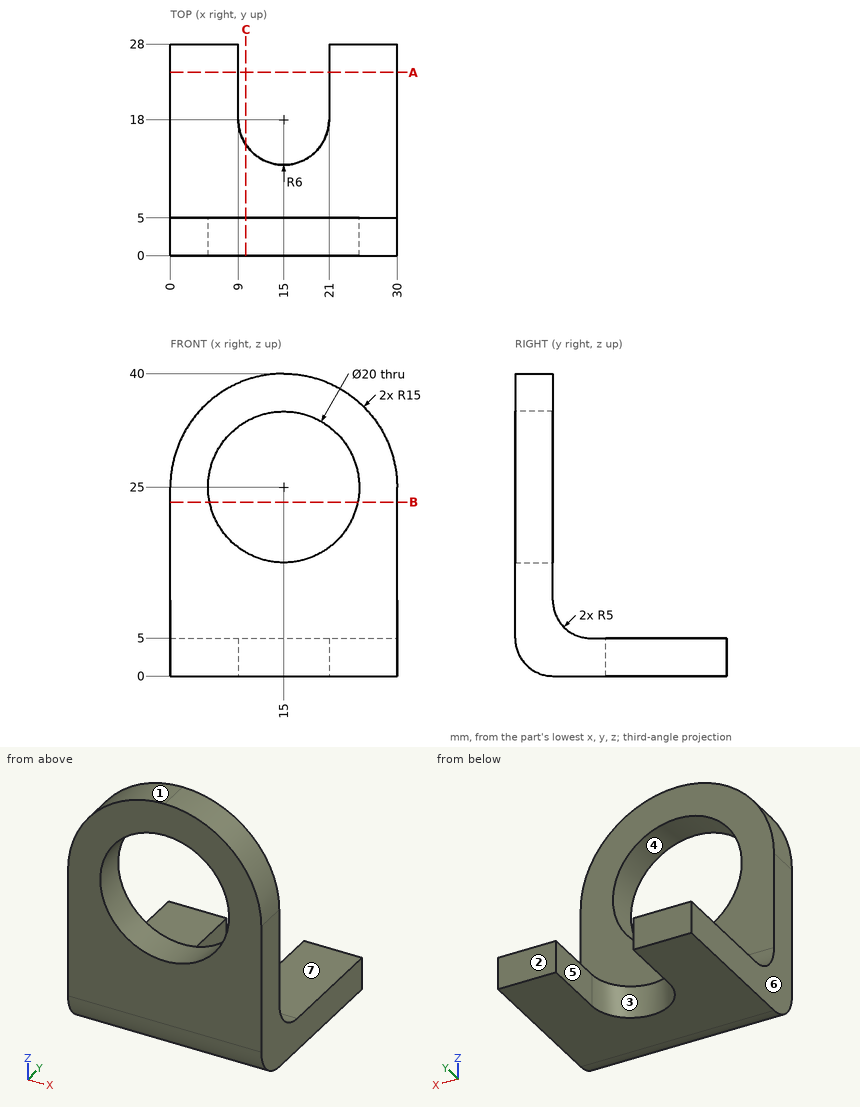
Here's the drawing with two shaded views (mm, measured from the low corner). I have some questions. A direction names the side the tool comes from. Give positions to 0.01 mm unless a question says otherwise; leave off trailing zeros. Write each loop counter-clockwise with the first axis right and the second up, starting at its lowest first coordinate (ties: lowest second). Pieces come first, ordered by that corner, then holes. Notation, with made-up numbers: (-40, 80.5) -> (-1, 80.5) arc R12 cw to (-1, 90.5) -> close; hole circle Ø3 at (81.5, -30). An arc over 180 degrees is marked (long way). Answer as a JSON object with one key per item and string values. Group by question number.
Item 1: I'm going to push flat-ended pins straight in: P1, Ø5.5, axis at x = 13.5, y = 15, coming from the +Z side; P2, Ø12, axis at x = 23.5, y = 9.5, coming from the +Z side. Where does each tip first touch, or does it pass through?
Item 2: Suppose I cut it at C-C (x = 10). Please give me the cut outline in (y, z), plus the area to 3 significant figures.
Item 3: Suppose I cut it at A-A (y = 24.25). Please give me the cut outline in (x, z), plus the area to 3 significant figures.
Item 4: We'd pull the mould along X, two halves only. Please class the marked faces 1, 2, 3 and 4: +X half, -X half, draft (parallel to the pull), parting line (faces both ways), or undercut.
Item 5: Suppose I cut it at B-B (z = 23). Please give me the cut outline in (x, y).
Item 6: Please list where these lines run through material, in increasing order: line 1 (Y direction, x = 27, z = 10); line 2 (X direction, y = 2.5, z = 34); line 3 (X direction, y = 4, z = 20.5). Write a range as [from, to].
Item 7: For the marked faces 5, 6 and 7, which set-ups out of +Z, -Z, +X, -X, +Y, -Y let a thin tool reach every point of the face, with its end or its side?
Findings:
{
 "1": {"P1": "stops at z = 5", "P2": "stops at z = 39.3"},
 "2": {"outline": "(0, 5) arc R5 ccw to (5, 0) -> (14.68, 0) -> (14.68, 5) -> (10, 5) arc R5 cw to (5, 10) -> (5, 16.34) -> (0, 16.34) -> close; (0, 33.66) -> (5, 33.66) -> (5, 39.14) -> (0, 39.14) -> close", "area": "158 mm²"},
 "3": {"outline": "(0, 0) -> (9, 0) -> (9, 5) -> (0, 5) -> close; (21, 0) -> (30, 0) -> (30, 5) -> (21, 5) -> close", "area": "90.0 mm²"},
 "4": {"face 1": "-X half", "face 2": "draft", "face 3": "undercut", "face 4": "undercut"},
 "5": {"outline": "(0, 0) -> (5.2, 0) -> (5.2, 5) -> (0, 5) -> close; (24.8, 0) -> (30, 0) -> (30, 5) -> (24.8, 5) -> close"},
 "6": {"line 1": "y = [0, 5]", "line 2": "x = [3, 10.64], [19.36, 27]", "line 3": "x = [0, 6.07], [23.93, 30]"},
 "7": {"face 5": "+Z, -Z, +Y", "face 6": "+Z, -Z, -X, +Y, -Y", "face 7": "+Z, +X, -X, +Y"}
}
